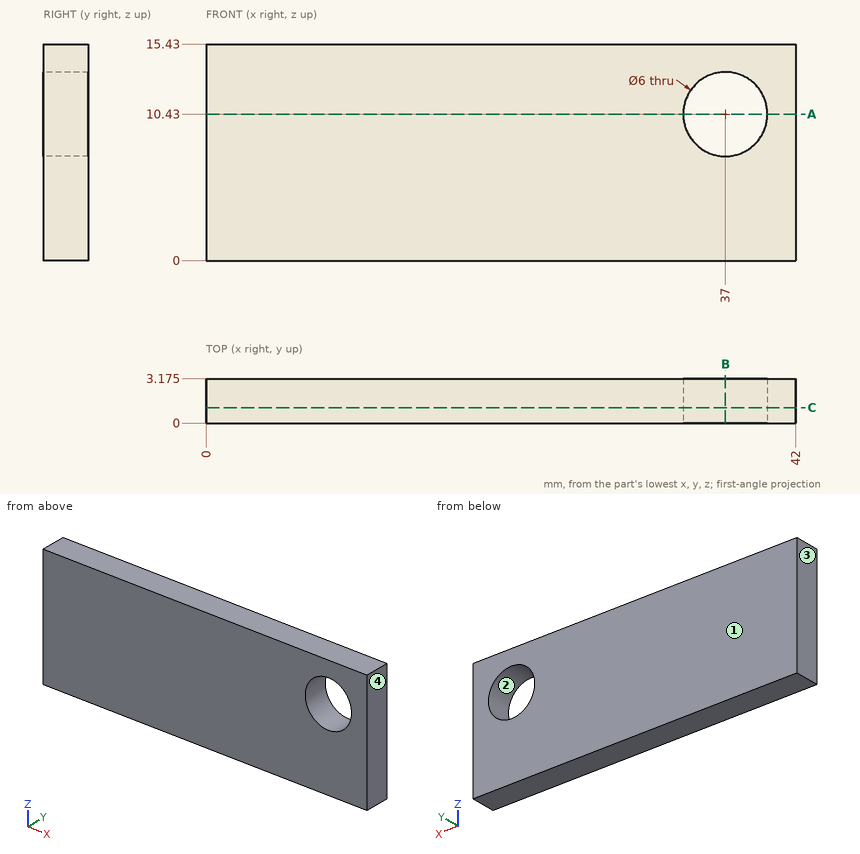
Study the drawing (mm; zero at the part's minimum x, y, z) and answer. Coordinates: 2 decimals unless noted, no trailing zeros. Loops run counter-clockwise (first coordinate to the right, second up) from the corner with the lowest first, then second, coordinate; pieces in that order, holes last. Notation, with made-up numbers: M -17.75,57 L 25.25,57 A20 ccw 25.25,88 Z; hole C 73.5,68.5 d7. An arc over 180 degrees is marked long. Answer as a JSON object with one key per item and string values. Group by question number.
Item 1: Determine the mould class of the marked faces 1, 2, 3 and 4 for opening direction X: +X half, -X half, draft (parallel to the pull), parting line (faces both ways), or undercut.
Item 2: This flat-tipped pin is pushed along its axis until it touches: P1, Ø1.5, axis at y = 2, z = 2, coming from the -X side. Where does it stop, or does it pass through?
Item 3: Section A-A (z = 10.43) is taken. Write down the section's boundary in (x, y) (3 decimals), and give its area (3 significant figures).
Item 4: Section C-C (y = 1.1) is taken. Write down the section's boundary in (x, z), and give its area (3 significant figures).
Item 5: Consider L1, parallel to X at y = 1.6, z = 10.43; L2, parallel to Z at x = 37, y = 2.1; L3, parallel to X at y = 3, z = 9.75. Determine where each line is inside the solid, lowest interval first.
Item 6: Section B-B (x = 37) is taken. Write down the section's boundary in (y, z) (3 decimals).
Solved:
{
 "1": {"face 1": "draft", "face 2": "undercut", "face 3": "-X half", "face 4": "+X half"},
 "2": {"P1": "stops at x = 0"},
 "3": {"outline": "M 0,0 L 34,0 L 34,3.175 L 0,3.175 Z; M 40,0 L 42,0 L 42,3.175 L 40,3.175 Z", "area": "114 mm2"},
 "4": {"outline": "M 0,0 L 42,0 L 42,15.43 L 0,15.43 Z; hole C 37,10.43 d6", "area": "620 mm2"},
 "5": {"L1": "x = 0 to 34, 40 to 42", "L2": "z = 0 to 7.43, 13.43 to 15.43", "L3": "x = 0 to 34.08, 39.92 to 42"},
 "6": {"outline": "M 0,0 L 3.175,0 L 3.175,7.43 L 0,7.43 Z; M 0,13.43 L 3.175,13.43 L 3.175,15.43 L 0,15.43 Z"}
}
